```python
from build123d import *

# Parameters (mm, degrees)
SKETCH1_W            = 220
SKETCH1_H            = 150
BOSS_EXTRUDE1_DEPTH  = 3.175
M3_CLEARANCE_HOLE1_D = 3.6
SKETCH4_W            = 10
SKETCH4_H            = 10
BOSS_EXTRUDE2_DEPTH  = 3.175
FILLET2_R            = 1.5
SKETCH5_W            = 200
SKETCH5_H            = 32
CUT_EXTRUDE1_DEPTH   = 4.175
FILLET3_R            = 5


with BuildPart() as part:
    # Sketch1 → Boss-Extrude1 (new body)
    with BuildSketch(Plane.XY):
        Rectangle(SKETCH1_W, SKETCH1_H)
    extrude(amount=BOSS_EXTRUDE1_DEPTH)

    # M3 Clearance Hole1 (through all)
    with Locations(Plane.XY.offset(3.175)):
        with Locations((0, 0), (-80, 70), (80, 70), (0, 70), (-105, 55), (-105, 0), (-105, -55), (-80, -70), (0, -70), (80, -70), (105, -55), (105, 0), (105, 55)):
            Hole(M3_CLEARANCE_HOLE1_D / 2)

    # Sketch4 → Boss-Extrude2 (add, through all)
    with BuildSketch(Plane.XY.offset(3.175)):
        Rectangle(SKETCH4_W, SKETCH4_H)
    extrude(amount=-BOSS_EXTRUDE2_DEPTH)

    # Fillet2
    fillet2_edges = [part.edges().sort_by_distance(p)[0] for p in [
        (-110, -75, 1.5875),
        (-110, 75, 1.5875),
        (110, 75, 1.5875),
        (110, -75, 1.5875),
    ]]
    fillet(fillet2_edges, radius=FILLET2_R)

    # Sketch5 → Cut-Extrude1 (cut, through all)
    with BuildSketch(Plane.XY.offset(3.175)):
        with Locations((0, -49)):
            Rectangle(SKETCH5_W, SKETCH5_H)
    extrude(amount=-CUT_EXTRUDE1_DEPTH, mode=Mode.SUBTRACT)

    # Fillet3
    fillet3_edges = [part.edges().sort_by_distance(p)[0] for p in [
        (100, -33, 1.5875),
        (100, -65, 1.5875),
        (-100, -65, 1.5875),
        (-100, -33, 1.5875),
    ]]
    fillet(fillet3_edges, radius=FILLET3_R)


solid = part.part
```
Read the model definition and answer for the solid it produces. Units are mm, in the model's axes. A direction names the side the tool comes from. Give positions to 0.01 mm unless a question says otherwise; leave off trailing zeros. Write each loop counter-clockwise with the first axis right and the second up, starting at its lowest first coordinate (ties: lowest second). Pieces come first, ordered by that corner, then holes. Notation, with made-up numbers: (33.5, -31) -> (43.5, -31) arc R19 ccw to (43.5, -16) -> close; hole circle Ø8 at (80, 52.25). An arc over 180 degrees is marked (long way). Answer in a Markdown table with one row per item.
1) Section B-B on z = 1.1 is taken. Count the separate pieces of the cut face and the enclosed holes in it, plus the area to 3 significant figures.
Results list:
| item | result |
|---|---|
| separate pieces | 1 |
| enclosed holes | 13 |
| area | 26,500 mm^2 |
2) Straight lines are drawn through the part: line 1 (Y direction, x = 105, z = 1.95); line 2 (Y direction, x = -80, z = 0.85); line 3 (X direction, y = -60, z = 2.5). For each, find the intervals that lie inside material, in ascending order. Write a range as [from, to].
Results list:
| item | result |
|---|---|
| line 1 | [-75, -56.8], [-53.2, -1.8], [1.8, 53.2], [56.8, 75] |
| line 2 | [-75, -71.8], [-68.2, -65], [-33, 68.2], [71.8, 75] |
| line 3 | [-110, -100], [100, 110] |
3) A tool of negligible diameter and unlimited length cuts with its end or side. For faces 3 (the cylindrical face through (99, -35, 2)), 4 (the flat face through (-2, 1, 0)), from which of +Z, -Z, +X, -X, +Y, -Y can it reach the whole face along a straight path? Write none if from no direction.
Results list:
| item | result |
|---|---|
| face 3 | +Z, -Z |
| face 4 | -Z, +X, -X, +Y, -Y |
4) Each of these flat-tipped pins is pushed along its axis until it touches: pin 1 Ø3 at (x, y) = (-7.5, 5) entering from -Z; pin 2 Ø2 at (x, y) = (-80, -70) entering from +Z. Where does it stop, or does it pass through?
Results list:
| item | result |
|---|---|
| pin 1 | z = 0 |
| pin 2 | through |
5) Determine the mould class of faces 1 (the cylindrical face through (98, -64, 2)), 2 (the flat face through (-2, 1, 3.175)) for opening direction X: released by +X, released by -X, zero draft, split by the parting line, or undercut.
Results list:
| item | result |
|---|---|
| face 1 | undercut |
| face 2 | zero draft |
6) Section A-A on x = -90.5 is taken. Give the vertices of the cut face in (y, z) (3 decimals).
Results list:
| item | result |
|---|---|
| outline | (-75, 0) -> (-65, 0) -> (-65, 3.175) -> (-75, 3.175) -> close; (-33, 0) -> (75, 0) -> (75, 3.175) -> (-33, 3.175) -> close |
